Verification items for the finished model (mm, model axes). A direction names the side the tool comes from. Coordinates: 2 decimals unless noted, no trailing zeros. Write each loop counter-clockwise with the first axis right and the second up, starting at its lowest first coordinate (ties: lowest second). Pieces come first, ordered by that corner, then holes. Notation, with made-up numbers: M 17.25,32.5 L 44.25,32.5 A12 cw 44.25,41.5 Z; hole C 17.25,47.5 d9. An arc over 180 degrees is marked long. One line per item, written item: value.
```python
from build123d import *

# Parameters (mm, degrees)
F1_DEPTH  = 7.62
F2_W      = 50.8
F2_H      = 14.000721
F3_DEPTH  = 1.27
F4_R      = 4.215081
F5_DEPTH  = 2.54
F6_W      = 40.64
F6_H      = 97.759279
F7_DEPTH  = 5.08
F8_R      = 5.08
F10_DEPTH = 1.27
F12_D     = 6.35


with BuildPart() as f1:
    # F0 (on Front) → F1 (new body)
    with BuildSketch(Plane.XZ):
        with BuildLine():
            Line((-7.261533, 95.628948), (-58.061533, 95.628948))
            ThreePointArc((-58.061533, 95.628948), (-67.041789, 91.909204), (-70.761533, 82.928948))
            Line((-70.761533, 82.928948), (-70.761533, -44.071052))
            ThreePointArc((-70.761533, -44.071052), (-67.041789, -53.051308), (-58.061533, -56.771052))
            Line((-58.061533, -56.771052), (-7.261533, -56.771052))
            ThreePointArc((-7.261533, -56.771052), (1.718724, -53.051308), (5.438467, -44.071052))
            Line((5.438467, -44.071052), (5.438467, 82.928948))
            ThreePointArc((5.438467, 82.928948), (1.718724, 91.909204), (-7.261533, 95.628948))
        make_face()
    extrude(amount=F1_DEPTH)

    # F2 (on face) → F3 (cut)
    with BuildSketch(Plane(origin=(0, 0, 0), x_dir=(-1, 0, 0), z_dir=(0, 1, 0))):
        with BuildLine():
            Line((7.261533, 68.928227), (7.261533, 82.928948))
            ThreePointArc((7.261533, 82.928948), (0.261172, 75.928588), (7.261533, 68.928227))
        make_face()
        with Locations((32.661533, 75.928587)):
            Rectangle(F2_W, F2_H)
        with BuildLine():
            ThreePointArc((58.061533, 68.928227), (65.061893, 75.928588), (58.061533, 82.928948))
            Line((58.061533, 82.928948), (58.061533, 68.928227))
        make_face()
    extrude(amount=-F3_DEPTH, mode=Mode.SUBTRACT)

    # F4 (on face) → F5 (join)
    with BuildSketch(Plane(origin=(0, -1.27, 0), x_dir=(-1, 0, 0), z_dir=(0, 1, 0))):
        with Locations((9.840052, 75.786227)):
            Circle(F4_R)
    extrude(amount=F5_DEPTH)

    # F6 (on face) → F7 (join)
    with BuildSketch(Plane(origin=(0, 0, 0), x_dir=(-1, 0, 0), z_dir=(0, 1, 0))):
        with Locations((32.661533, 17.508588)):
            Rectangle(F6_W, F6_H)
    extrude(amount=F7_DEPTH)

    # F8
    f8_edges = [f1.edges().sort_by_distance(p)[0] for p in [
        (-12.341533, 2.54, 66.388227),
        (-52.981533, 2.54, 66.388227),
        (-52.981533, 2.54, -31.371052),
        (-12.341533, 2.54, -31.371052),
    ]]
    fillet(f8_edges, radius=F8_R)

    # F9 (on face) → F10 (cut)
    with BuildSketch(Plane.XZ.offset(7.62)):
        with BuildLine():
            Line((-12.341533, 90.548948), (-52.981533, 90.548948))
            ThreePointArc((-52.981533, 90.548948), (-61.961789, 86.829204), (-65.681533, 77.848948))
            Line((-65.681533, 77.848948), (-65.681533, -38.991052))
            ThreePointArc((-65.681533, -38.991052), (-61.961789, -47.971308), (-52.981533, -51.691052))
            Line((-52.981533, -51.691052), (-12.341533, -51.691052))
            ThreePointArc((-12.341533, -51.691052), (-3.361276, -47.971308), (0.358467, -38.991052))
            Line((0.358467, -38.991052), (0.358467, 77.848948))
            ThreePointArc((0.358467, 77.848948), (-3.361276, 86.829204), (-12.341533, 90.548948))
        make_face()
    extrude(amount=-F10_DEPTH, mode=Mode.SUBTRACT)

    # F12 (through all)
    with Locations(Plane.XZ.offset(6.35)):
        with Locations((-34.155931, 13.220405)):
            Hole(F12_D / 2)


solid = f1.part
```
Item 1: Go/stop test with flat-tipped pins: P1, Ø2.5, axis at y = 1.5, z = 16, coming from the +X side; P2, Ø15.5, axis at x = -38, z = 77, coming from the +Y side; P3, Ø5.5, axis at x = -34.16, z = 13.22, coming from the +Y side; P4, Ø2.5, axis at x = -36, y = 1.5, coming from the -Z side. Record where each tip stops, or that it passes through.
The answers:
P1: stops at x = -12.34
P2: stops at y = 0
P3: passes through
P4: stops at z = -31.37
Item 2: Draft check along Z on faces 1 (the face through (-70.762, -4, 20)), 2 (the face through (-3.46, -6.99, -48.07)), 3 (the face through (-66.94, -3.76, 92.01)). Enter one of: released by +Z, released by -Z, zero draft, split by the parting line, or undercut.
The answers:
face 1: zero draft
face 2: undercut
face 3: released by +Z
Item 3: Cross-section at C-C, the plane y = 3.25. Enter the section's corners in (x, z) (3 decimals).
The answers:
outline: M -52.982,-26.291 A5.08 ccw -47.902,-31.371 L -17.422,-31.371 A5.08 ccw -12.342,-26.291 L -12.342,61.308 A5.08 ccw -17.422,66.388 L -47.902,66.388 A5.08 ccw -52.982,61.308 Z; hole C -34.156,13.22 d6.35
Item 4: Cross-section at A-A, the plane z = 52. Enter the section's corners in (x, y).
The answers:
outline: M -70.76,-7.62 L -65.68,-7.62 L -65.68,-6.35 L 0.36,-6.35 L 0.36,-7.62 L 5.44,-7.62 L 5.44,0 L -12.34,0 L -12.34,5.08 L -52.98,5.08 L -52.98,0 L -70.76,0 Z
Item 5: Scan lines: line 1 (Z direction, x = -11.5, y = -6.75); line 2 (Y direction, x = 0, z = -6); line 3 (Y direction, x = -45, z = 43). Record each from-to range of solid material in increasing order.
The answers:
line 1: z = -56.77 to -51.66, 90.52 to 95.63
line 2: y = -6.35 to 0
line 3: y = -6.35 to 5.08
Item 6: Cross-section at D-D, the plane z = -34. Enter the section's corners in (x, y), and give its area (3 significant figures).
The answers:
outline: M -70.76,-7.62 L -65.68,-7.62 L -65.68,-6.35 L 0.36,-6.35 L 0.36,-7.62 L 5.44,-7.62 L 5.44,0 L -70.76,0 Z
area: 497 mm²
Item 7: Cross-section at B-B, the plane x = -22. Enter the section's corners in (y, z).
The answers:
outline: M -7.62,-56.77 L 0,-56.77 L 0,-31.37 L 5.08,-31.37 L 5.08,66.39 L 0,66.39 L 0,68.93 L -1.27,68.93 L -1.27,82.93 L 0,82.93 L 0,95.63 L -7.62,95.63 L -7.62,90.55 L -6.35,90.55 L -6.35,-51.69 L -7.62,-51.69 Z
Item 8: Access from +Z, -Z, +X, -X, +Y, -Y to the whole of each face (thin tool, end or side, straight path). Record for faces 4 (the face through (-0.263, -0.626, 76.083)), 5 (the face through (-61.86, -6.99, 86.93)), 6 (the face through (-13.79, 2.576, -29.843)).
The answers:
face 4: +Y
face 5: -Y
face 6: -Z, +X, +Y
